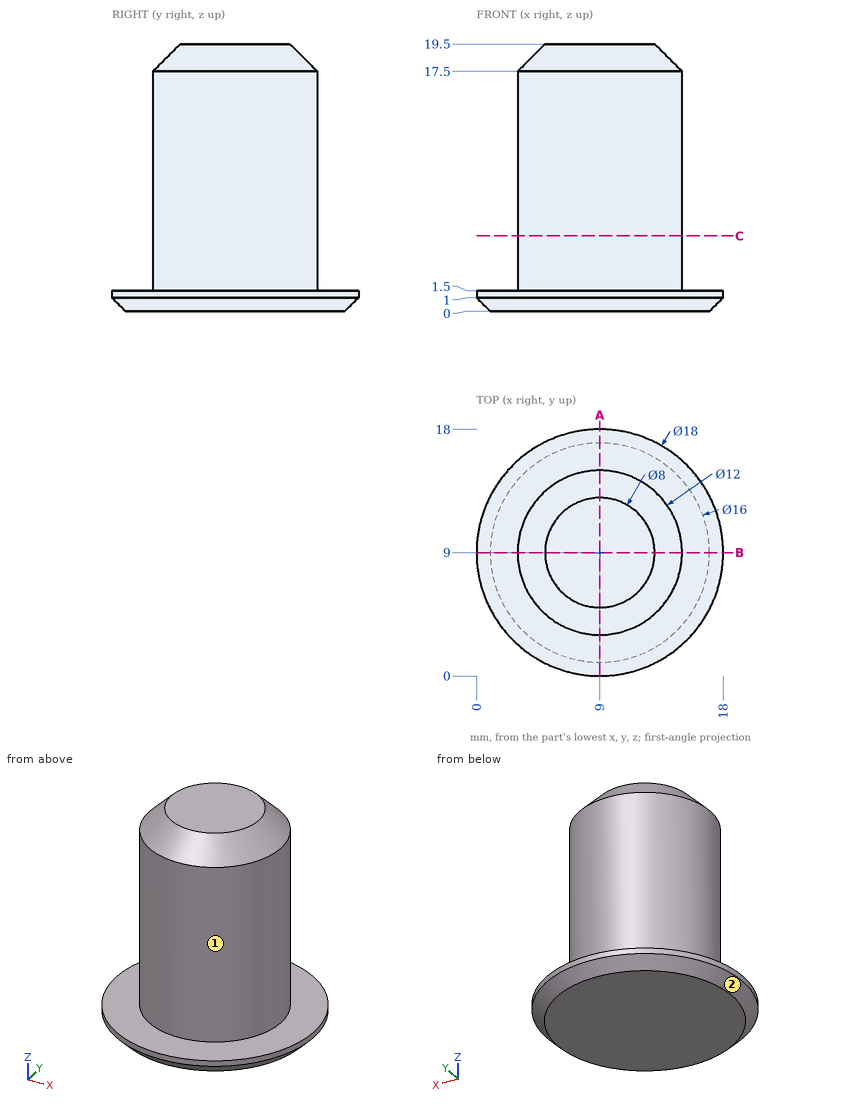
Answer from the drawing. Dimensions are ordinates in mm from the lowest x, y and z of the part. A direction names the side the tool comes from. Round coordinates to 2 decimals unless told otherwise and drop trailing zeros. Loops run counter-clockwise (first coordinate to the right, second up) from the corner with the lowest first, then second, coordinate; pieces in that order, holes last. Notation, with made-up numbers: M -21,-24 L 9,-24 A27 ccw 9,2 Z; hole C -9,16.25 d8. An arc over 180 degrees is marked long. One line per question, with ' | ' between items. Start each with the question number.
(1) A cutting plane is placed at C-C on z = 5.5. Write down the section's boundary in (x, y), plus the area to 3 significant figures.
(2) A flat-ended cylindrical pin translates along its axis: pin 1 Ø8 at (x, z) = (3, 8) entering from +Y. Find the tip coordinate at first contact, or state that the pin passes through.
(3) A cutting plane is placed at A-A on x = 9. Write down the section's boundary in (y, z).
(4) A tool of negligible diameter and unlimited length cuts with its end or side. For the marked faces 1 and 2, from which of +Z, -Z, +X, -X, +Y, -Y can it reach the whole face along a straight path? Write none if from no direction.
(5) Find the intervals of material crossed by line 1 (Z direction, x = 15.25, y = 6); line 2 (Y direction, x = 5.75, z = 10.5); line 3 (Z direction, x = 6, y = 11.75), in increasing order.
Geometry check:
1) outline: C 9,9 d12 | area: 113 mm²
2) pin 1: stops at y = 14.66
3) outline: M 0,1 L 1,0 L 17,0 L 18,1 L 18,1.5 L 15,1.5 L 15,17.5 L 13,19.5 L 5,19.5 L 3,17.5 L 3,1.5 L 0,1.5 Z
4) face 1: +Z | face 2: -Z
5) line 1: z = 0 to 1.5 | line 2: y = 3.96 to 14.04 | line 3: z = 0 to 19.43
